Input: part model. Units: mm. Frame: model coordinates. Face numbers are marked on the shaded views. Round coordinates to 2 decimals unless told otherwise and drop trailing zeros. Order: outer loops, then holes, each group sorted by start corner. A loop starts at its lowest first (then second) coordinate and runs counter-clockwise, first axis right, second up. Notation, with made-up numbers: (-17.75, 18) -> (-8.75, 18) arc R25 ccw to (-8.75, 51) -> close; hole circle Ø10 at (47, -7). An arc over 180 degrees is marked (long way). Use a Markdown table: item, result.
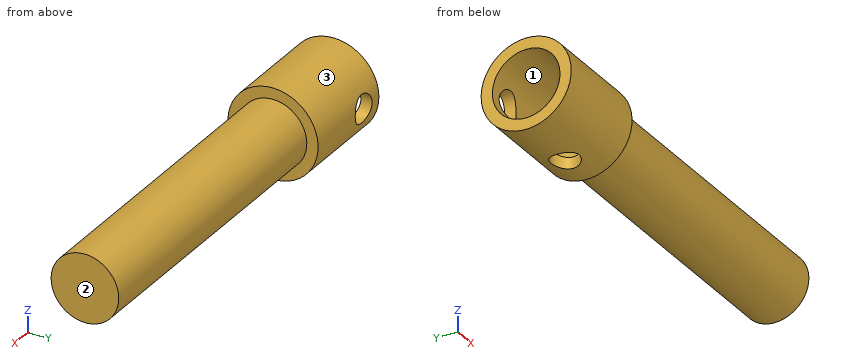
from build123d import *

# Parameters (mm, degrees)
F3_R     = 1.5
F5_DEPTH = 4.801
F4_R     = 1.5
F6_DEPTH = 4.801


with BuildPart() as f2:
    # F1 (on Front) → F2 (revolve)
    with BuildSketch(Plane.XZ):
        Polygon((0, 4.8), (0, 3.6), (9.6, 3.6), (9.6, 2.4), (18.6, 2.4), (43, 2.4), (43, 0), (44.2, 0), (44.2, 3.6), (18.6, 3.6), (10.8, 3.6), (10.8, 4.8), align=None)
    revolve(axis=Axis((43.6, 0, 0), (1, 0, 0)))

    # F3 (on Front) → F5 (cut, through all)
    with BuildSketch(Plane.XZ):
        with Locations((2.7, 0)):
            Circle(F3_R)
    extrude(amount=-F5_DEPTH, mode=Mode.SUBTRACT)

    # F4 (on Top) → F6 (cut, through all)
    with BuildSketch(Plane.XY):
        with Locations((6.9, 0)):
            Circle(F4_R)
    extrude(amount=-F6_DEPTH, mode=Mode.SUBTRACT)


solid = f2.part
1) Cut plane D-D on y = 4. Return loops of the section in (x, z), and give its area (3 significant figures).
Results found:
| item | result |
|---|---|
| outline | (0, -2.65) -> (10.8, -2.65) -> (10.8, 2.65) -> (0, 2.65) -> close; hole circle Ø3 at (2.7, 0) |
| area | 50.2 mm² |
2) Cut plane B-B on y = 0. Return loops of the section in (x, z), and give its area (3 significant figures).
Results found:
| item | result |
|---|---|
| outline | (0, -4.8) -> (5.4, -4.8) -> (5.4, -3.6) -> (0, -3.6) -> close; (0, 3.6) -> (9.6, 3.6) -> (9.6, 2.4) -> (43, 2.4) -> (43, -2.4) -> (9.6, -2.4) -> (9.6, -3.6) -> (8.4, -3.6) -> (8.4, -4.8) -> (10.8, -4.8) -> (10.8, -3.6) -> (44.2, -3.6) -> (44.2, 3.6) -> (10.8, 3.6) -> (10.8, 4.8) -> (0, 4.8) -> close |
| area | 111 mm² |
3) Pin query (flat end, axial travel): pin 1 Ø3 at (x, y) = (16, 4) entering from +Z; pin 2 Ø1.4 at (y, z) = (0, -0.5) entering from -X; pin 3 Ø3 at (y, z) = (-4, -0.5) entering from -X; pin 4 Ø5 at (x, z) = (29.5, -0.5) entering from +Y. Return the tip coordinate at first contact, or that it passes through.
Results found:
| item | result |
|---|---|
| pin 1 | stops at z = 2.59 |
| pin 2 | stops at x = 43 |
| pin 3 | stops at x = 0 |
| pin 4 | stops at y = 3.6 |
4) Line query: L1, parallel to Z at x = 25, y = 0; L2, parallel to X at y = 0, z = -4.25; L3, parallel to X at y = 4.25, z = 0. Output: solid intervals per line, ascending. Write a range as [from, to].
Results found:
| item | result |
|---|---|
| L1 | z = [-3.6, -2.4], [2.4, 3.6] |
| L2 | x = [0, 5.4], [8.4, 10.8] |
| L3 | x = [0, 1.2], [4.2, 10.8] |
5) Cut plane C-C on x = 22. Return loops of the section in (y, z), and give its area (3 significant figures).
Results found:
| item | result |
|---|---|
| outline | circle Ø7.2 at (0, 0); hole circle Ø4.8 at (0, 0) |
| area | 22.6 mm² |
6) Cut plane A-A on z = 0. Return loops of the section in (x, y), and give its area (3 significant figures).
Results found:
| item | result |
|---|---|
| outline | (0, -4.8) -> (10.8, -4.8) -> (10.8, -3.6) -> (44.2, -3.6) -> (44.2, 3.6) -> (10.8, 3.6) -> (10.8, 4.8) -> (4.2, 4.8) -> (4.2, 3.6) -> (9.6, 3.6) -> (9.6, 2.4) -> (43, 2.4) -> (43, -2.4) -> (9.6, -2.4) -> (9.6, -3.6) -> (0, -3.6) -> close; (0, 3.6) -> (1.2, 3.6) -> (1.2, 4.8) -> (0, 4.8) -> close |
| area | 111 mm² |
7) Pull-direction query (Y, two-part tool) for the marked faces 1, 2 and 3; classes: +Y half, -Y half, draft (parallel to the pull), parting line (faces both ways), or undercut.
Results found:
| item | result |
|---|---|
| face 1 | undercut |
| face 2 | draft |
| face 3 | parting line |
